Model file for the job. Use its own axes, mm. Face numbers are marked on the shaded views. A direction names the side the tool comes from. Round coordinates to 2 decimals unless told otherwise and drop trailing zeros. Order: outer loops, then holes, each group sorted by start corner. A loop starts at its lowest first (then second) coordinate and runs counter-clockwise, first axis right, second up. Notation, with made-up numbers: (68.25, 35.25) - (124.25, 35.25) arc R20 cw to (124.25, 61.25) - close; hole circle Ø9 at (69.25, -25). An arc over 180 degrees is marked (long way). Put each result on its own line as item: value. Start each with the question number.
Item 1: Saw through at A-A on x = 26.4. List the corners of the cut face in (y, z), plus the area to 3 significant figures.
Item 2: Pin check, flat tips, straight feed: pin 1 Ø5 at (y, z) = (-5, 20.5) entering from -X; pin 2 Ø1.5 at (y, z) = (2.5, 27.5) entering from +X; pin 3 Ø5 at (y, z) = (-0.5, 34.5) entering from +X; pin 4 Ø4 at (x, y) = (26.4, 6) entering from -Z. Stop position of each tip, or through.
Item 3: Saw through at D-D on y = 1.25. List the corners of the cut face in (x, z), plus the area to 3 significant figures.
Item 4: Mould opens along Z. For the marked faces 6, 7 and 8 say: pulls with the +Z half, pulls with the -Z half, needs draft (parallel to the pull), parting line crosses it, or undercut.
Item 5: Saw through at C-C on x = -26.4. List the corners of the cut face in (y, z).
Item 6: Probe probe 1 along Y at (x, z) = (26.4, 29.25); probe 2 along Z at (x, y) = (24.5, 3.25); probe 3 along X at (y, z) = (-10, 22.5). List the from-to ranges inside material, lowest first.
Item 7: Saw through at B-B on y = 6. List the corners of the cut face in (x, z), plus the area to 3 significant figures.
Item 8: Which spindle directions (+Z, -Z, +X, -X, +Y, -Y) get a long thin tool onto all of the face, cutting with end or side? Do the marked faces 1, 2, 3, 4 and 5. Say none if no direction does.
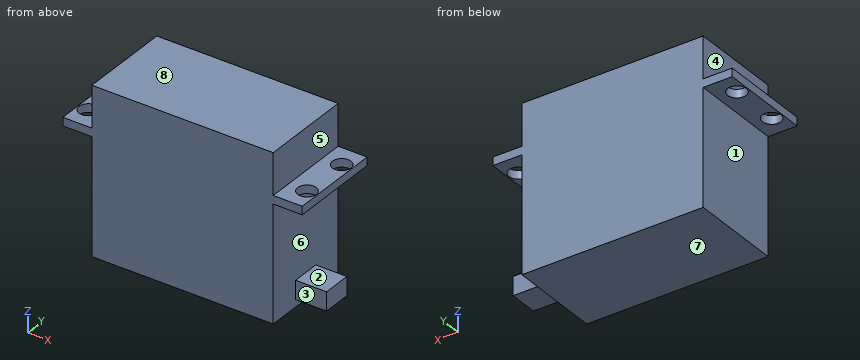
```python
from build123d import *

# Parameters (mm, degrees)
F0_W     = 21.9
F0_H     = 22.4
F1_DEPTH = 40
F2_START = 28
F0_W_2   = 7
F2_DEPTH = 2
F3_D     = 4.5
F5_W     = 7
F5_H     = 4.5
F6_DEPTH = 7.5


with BuildPart() as f1:
    # F0 (on Top) → F1 (new body)
    with BuildSketch(Plane.XY):
        with Locations((10.95, 0)):
            Rectangle(F0_W, F0_H)
    extrude(amount=F1_DEPTH)

    # F0 (on Top) → F2 (join)
    with BuildSketch(Plane.XY.offset(F2_START)):
        with Locations((25.4, 0)):
            Rectangle(F0_W_2, F0_H)
    extrude(amount=F2_DEPTH)

    # F3 (through all)
    with Locations(Plane(origin=(0, 0, 0), x_dir=(1, 0, 0), z_dir=(0, 0, -1))):
        with Locations((26.4, 6), (26.4, -6)):
            Hole(F3_D / 2)

    # F4: F1 across face


with BuildPart() as f1_1:
    add(f1.part)
    add(f1.part.mirror(Plane(origin=(0, 0, 20), x_dir=(0, -1, 0), z_dir=(-1, 0, 0))))

    # F5 (on face) → F6 (join)
    with BuildSketch(Plane.YZ.offset(21.9)):
        with Locations((0, 4)):
            Rectangle(F5_W, F5_H)
    extrude(amount=F6_DEPTH)


solid = f1_1.part
```
Results found:
1. outline: (-11.2, 28) - (-8.25, 28) - (-8.25, 30) - (-11.2, 30) - close; (-3.75, 28) - (3.75, 28) - (3.75, 30) - (-3.75, 30) - close; (-3.5, 1.75) - (3.5, 1.75) - (3.5, 6.25) - (-3.5, 6.25) - close; (8.25, 28) - (11.2, 28) - (11.2, 30) - (8.25, 30) - close
1. area: 58.3 mm²
2. pin 1: stops at x = -21.9
2. pin 2: stops at x = 28.9
2. pin 3: stops at x = 21.9
2. pin 4: passes through
3. outline: (-28.9, 28) - (-21.9, 28) - (-21.9, 0) - (21.9, 0) - (21.9, 1.75) - (29.4, 1.75) - (29.4, 6.25) - (21.9, 6.25) - (21.9, 28) - (28.9, 28) - (28.9, 30) - (21.9, 30) - (21.9, 40) - (-21.9, 40) - (-21.9, 30) - (-28.9, 30) - close
3. area: 1,810 mm²
4. face 6: undercut
4. face 7: pulls with the -Z half
4. face 8: pulls with the +Z half
5. outline: (-11.2, 28) - (-8.25, 28) - (-8.25, 30) - (-11.2, 30) - close; (-3.75, 28) - (3.75, 28) - (3.75, 30) - (-3.75, 30) - close; (8.25, 28) - (11.2, 28) - (11.2, 30) - (8.25, 30) - close
6. probe 1: y = -11.2 to -8.25, -3.75 to 3.75, 8.25 to 11.2
6. probe 2: z = 1.75 to 6.25, 28 to 30
6. probe 3: x = -21.9 to 21.9
7. outline: (-28.9, 28) - (-28.65, 28) - (-28.65, 30) - (-28.9, 30) - close; (-24.15, 28) - (-21.9, 28) - (-21.9, 0) - (21.9, 0) - (21.9, 28) - (24.15, 28) - (24.15, 30) - (21.9, 30) - (21.9, 40) - (-21.9, 40) - (-21.9, 30) - (-24.15, 30) - close; (28.65, 28) - (28.9, 28) - (28.9, 30) - (28.65, 30) - close
7. area: 1,760 mm²
8. face 1: -Z, -X, +Y, -Y
8. face 2: +X, +Y, -Y
8. face 3: -Z, +X, -Y
8. face 4: +Z, -X, +Y, -Y
8. face 5: +Z, +X, +Y, -Y
